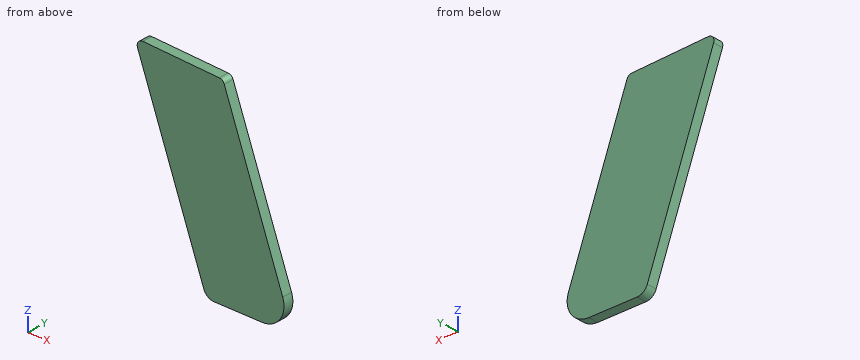
from build123d import *

# Parameters (mm, degrees)
F1_DEPTH = 5.842
F2_R     = 6.35
F3_R     = 12.7
F6_DEPTH = 25.4
F7_R     = 3.175


# Not quite as in the source:
# - a length typed as a fraction of an inch, garbled in the dataset ("3 / 203.2 mm" for 3/8 in), is restored


with BuildPart() as f1:
    # F0 (on Front) → F1 (new body)
    with BuildSketch(Plane.XZ):
        Polygon((50.8, 0), (0, 0), (55.4690637022, -152.4), (106.2690637022, -152.4), align=None)
    extrude(amount=F1_DEPTH)

    # F2
    f2_edges = [f1.edges().sort_by_distance(p)[0] for p in [
        (55.469064, -2.921, -152.4),
        (50.8, -2.921, 0),
        (0, -2.921, 0),
    ]]
    fillet(f2_edges, radius=F2_R)

    # F3
    f3_edges = [f1.edges().sort_by_distance(p)[0] for p in [
        (106.269064, -2.921, -152.4),
    ]]
    fillet(f3_edges, radius=F3_R)

    # F5 (on face) → F6 (cut)
    with BuildSketch(Plane.XZ.offset(5.842)):
        Polygon((109.8922565579, 0), (-38.8115942478, 0), (-38.8115942478, -34.925), (109.8922565579, -41.275), align=None)
    extrude(amount=-F6_DEPTH, mode=Mode.SUBTRACT)

    # F7
    f7_edges = [f1.edges().sort_by_distance(p)[0] for p in [
        (65.127115, -2.921, -39.363424),
        (13.525097, -2.921, -37.159898),
    ]]
    fillet(f7_edges, radius=F7_R)


solid = f1.part
Design review of the part built by this model. Coordinates are the model's own, in mm. Give positions to 0.01 mm unless a question says otherwise; leave off trailing zeros. Write each loop counter-clockwise with the first axis right and the second up, starting at its lowest first coordinate (ties: lowest second). Pieces come first, ordered by that corner, then holes. Notation, with made-up numbers: M 23,66.25 L 30,66.25 A30 ccw 30,88.25 Z; hole C 37,25 d3. An arc over 180 degrees is marked long. Answer as a JSON object with one key per item and string values. Group by question number.
1) For line 1 along X through (y, z) = (-3.1, -79); line 2 along X through (y, z) = (-0.35, -112); line 3 along Z through (x, y) = (65, -5.3), list the stretches that pass through material, from the lowest coordinate up.
2) We need section B-B (x = 37.5). Give the boundary of the cut face in (y, z), and give its area (3 significant figures).
3) Clearance check with flat-ended pins moving along their axes: pin 1 Ø10 at (x, z) = (37, -93.5) entering from +Y; pin 2 Ø1.5 at (x, y) = (33, -4.5) entering from +Z; pin 3 Ø2 at (y, z) = (-3, -64.5) entering from -X. State where each tip first meets the part, or that it passes through.
4) We need section C-C (z = -97.5). Give the boundary of the cut face in (x, y), and give its area (3 significant figures).
5) We need section A-A (y = -4.55). Give the boundary of the cut face in (x, z) (3 decimals).
Answer key:
{
 "1": {"line 1": "x = 28.75 to 79.55", "line 2": "x = 40.76 to 91.56", "line 3": "z = -152.4 to -40.09"},
 "2": {"outline": "M -5.84,-103.03 L 0,-103.03 L 0,-38.18 L -5.84,-38.18 Z", "area": "379 mm²"},
 "3": {"pin 1": "stops at y = 0", "pin 2": "stops at z = -37.96", "pin 3": "stops at x = 23.11"},
 "4": {"outline": "M 35.49,-5.84 L 86.29,-5.84 L 86.29,0 L 35.49,0 Z", "area": "297 mm²"},
 "5": {"outline": "M 15.149,-41.62 L 53.948,-148.222 A6.35 ccw 59.915,-152.4 L 88.132,-152.4 A12.7 ccw 100.066,-135.356 L 65.853,-41.359 A3.175 ccw 63.005,-39.273 L 18.268,-37.362 A3.175 ccw Z"}
}
